Could you check a few things on this model? Use its own coordinates, in mm. Face numbers are marked on the shaded views. Round coordinates to 2 decimals unless told otherwise and drop trailing zeros. Write each loop counter-clockwise with the first axis right and the second up, starting at its lowest first coordinate (ties: lowest second). Pieces come first, ordered by that corner, then holes.
```python
from build123d import *

# Parameters (mm, degrees)
F1_DEPTH  = 15
F4_R      = 2.55
F2_R      = 2.655
F7_D      = 3.5
F8_F1_R   = 2
F9_W      = 2
F9_H      = 1
F9_W_2    = 1
F9_H_2    = 2
F10_DEPTH = 0.5


with BuildPart() as f1:
    # F0 (on Top) → F1 (new body)
    with BuildSketch(Plane.XY):
        Polygon((12.5, -3), (40, -3), (40, 3), (-40, 3), (-40, -3), (-12.5, -3), (-12.5, -1.75), (12.5, -1.75), align=None)
    extrude(amount=F1_DEPTH)

    # F4 (on offset) → F5 section 0
    with BuildSketch(Plane.XZ.offset(-0.8)):
        with Locations((-30, 7.5)):
            Circle(F4_R)
    # F2 (on face) → F5 section 1
    with BuildSketch(Plane.XZ.offset(3)):
        with Locations((-30, 7.5)):
            Circle(F2_R)
    loft(mode=Mode.SUBTRACT)

    # F2 (on face) → F6 section 0
    with BuildSketch(Plane.XZ.offset(3)):
        with Locations((30, 7.5)):
            Circle(F2_R)
    # F4 (on offset) → F6 section 1
    with BuildSketch(Plane.XZ.offset(-0.8)):
        with Locations((30, 7.5)):
            Circle(F4_R)
    loft(mode=Mode.SUBTRACT)

    # F7 (through all)
    with Locations(Plane.XZ.offset(-0.8)):
        with Locations((30, 7.5), (-30, 7.5)):
            Hole(F7_D / 2)

    # F8: fillet of radius 2 on 2 edges, made by hand

    # F8_f1
    f8_f1_edges = [f1.edges().sort_by_distance(p)[0] for p in [
        (26.25, -3, 0),
    ]]
    fillet(f8_f1_edges, radius=F8_F1_R)

    # F9 (on face) → F10 (cut)
    with BuildSketch(Plane.XY.offset(15)):
        with Locations((-31.5, 0)):
            Rectangle(F9_W, F9_H)
        with Locations((-30, 0)):
            Rectangle(F9_W_2, F9_H)
        with Locations((-28.5, 0)):
            Rectangle(F9_W, F9_H)
        with Locations((-30, 1.5)):
            Rectangle(F9_W_2, F9_H_2)
        with Locations((-30, -1.5)):
            Rectangle(F9_W_2, F9_H_2)
    extrude(amount=-F10_DEPTH, mode=Mode.SUBTRACT)


solid = f1.part
```
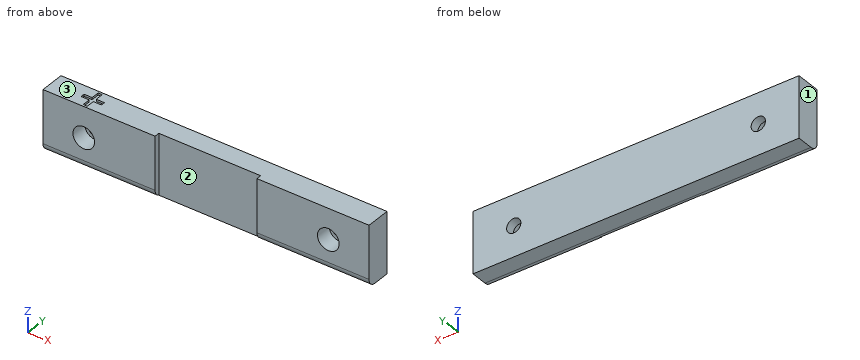
Q1. Imagine slicing it at C-C, the plane z = 7.5. Count the separate pieces of the cut face and the enclosed holes in it, then the cut area to 3 significant figures.
Q2. We'd pull the mould along X, two halves only. Please class the marked faces 1, 2 and 3: pulls with the +X half, pulls with the -X half, needs draft (parallel to the pull), parting line crosses it, or undercut.
Q3. Imagine slicing it at A-A, the plane y = 1.5. Write out the boundary of the cut face in (x, z), then the cut area to 3 significant figures.
Q4. Imagine slicing it at B-B, the plane x = 30. Write out the boundary of the cut face in (y, z) (3 decimals), then the cut area to 3 significant figures.
Q5. I'm going to push flat-ended pins straight in: pin 1 Ø4.5 at (x, z) = (-30, 7.5) entering from -Y; pin 2 Ø5.5 at (x, z) = (29, 7) entering from -Y. Where does each tip first touch, or does it pass through?
Q6. Imagine slicing it at D-D, the plane z = 11.5. Write out the boundary of the cut face in (x, y), then the cut area to 3 significant figures.
Q7. If I drill on L1, parallel to X at y = -2, z = 11.5; L2, parallel to Z at x = 30, y = 2.5; L3, parallel to Z at x = -30, y = 1.6, over which ranges is the centre line in solid material (lowest first)?
Results found:
1. separate pieces: 3
1. enclosed holes: 0
1. area: 394 mm2
2. face 1: pulls with the -X half
2. face 2: undercut
2. face 3: needs draft
3. outline: (-40, 0) - (40, 0) - (40, 15) - (-29.5, 15) - (-29.5, 14.5) - (-30.5, 14.5) - (-30.5, 15) - (-40, 15) - close; hole circle Ø3.5 at (-30, 7.5); hole circle Ø3.5 at (30, 7.5)
3. area: 1,180 mm2
4. outline: (-3, 2) arc R2 ccw to (-1, 0) - (3, 0) - (3, 5.75) - (0.8, 5.75) - (0.8, 4.95) - (-3, 4.845) - close; (-3, 10.155) - (0.8, 10.05) - (0.8, 9.25) - (3, 9.25) - (3, 15) - (-3, 15) - close
4. area: 61.7 mm2
5. pin 1: stops at y = 0.8
5. pin 2: stops at y = -3
6. outline: (-40, -3) - (-12.5, -3) - (-12.5, -1.75) - (12.5, -1.75) - (12.5, -3) - (40, -3) - (40, 3) - (-40, 3) - close
6. area: 449 mm2
7. L1: x = -40 to -12.5, 12.5 to 40
7. L2: z = 0 to 5.75, 9.25 to 15
7. L3: z = 0 to 5.75, 9.25 to 14.5
